```python
from build123d import *

# Parameters (mm, degrees)
SKETCH_1_R          = 2.9
EXTRUDE_3_DEPTH     = 1
EXTRUDE_6_DEPTH     = 47
CUT_EXTRUDE_START   = -1.3
CUT_EXTRUDE_1_DEPTH = 1.3
CUT_EXTRUDE_START_2 = -1.5
SKETCH_6_W          = 2.2
SKETCH_6_H          = 2.6
CUT_EXTRUDE_2_DEPTH = 1.5


with BuildPart() as part:
    # Эскиз1 → Бобышка-Вытянуть3 (new body)
    with BuildSketch(Plane(origin=(0, 0, 0), x_dir=(1, 0, 0), z_dir=(0, 1, 0))):
        with BuildLine():
            Line((-11.72321672, 11.668784432), (-11.72321672, 27.268784432))
            ThreePointArc((-11.72321672, 27.268784432), (-11.137430283, 28.682997994), (-9.72321672, 29.268784432))
            Line((-9.72321672, 29.268784432), (11.27678328, 29.268784432))
            ThreePointArc((11.27678328, 29.268784432), (12.690996842, 28.682997994), (13.27678328, 27.268784432))
            Line((13.27678328, 27.268784432), (13.27678328, 11.668784432))
            ThreePointArc((13.27678328, 11.668784432), (12.690996842, 10.254570869), (11.27678328, 9.668784432))
            Line((11.27678328, 9.668784432), (9.27678328, 9.668784432))
            Line((9.27678328, 9.668784432), (-9.72321672, 9.668784432))
            ThreePointArc((-9.72321672, 9.668784432), (-11.137430283, 10.254570869), (-11.72321672, 11.668784432))
        make_face()
        with Locations(Location((5.02678328, 15.968784432, 0), (0, 0, 270))):
            Circle(SKETCH_1_R, mode=Mode.SUBTRACT)
        with BuildLine():
            Line((-1.45321672, 26.968784432), (5.00678328, 26.968784432))
            ThreePointArc((5.00678328, 26.968784432), (6.187651604, 26.479652756), (6.67678328, 25.298784432))
            Line((6.67678328, 25.298784432), (6.67678328, 24.638784432))
            ThreePointArc((6.67678328, 24.638784432), (6.187651604, 23.457916107), (5.00678328, 22.968784432))
            Line((5.00678328, 22.968784432), (-1.45321672, 22.968784432))
            ThreePointArc((-1.45321672, 22.968784432), (-2.634085045, 23.457916107), (-3.12321672, 24.638784432))
            Line((-3.12321672, 24.638784432), (-3.12321672, 25.298784432))
            ThreePointArc((-3.12321672, 25.298784432), (-2.634085045, 26.479652756), (-1.45321672, 26.968784432))
        make_face(mode=Mode.SUBTRACT)
    extrude(amount=EXTRUDE_3_DEPTH)

    # Эскиз3 → Бобышка-Вытянуть6 (add)
    with BuildSketch(Plane(origin=(0, 1, 0), x_dir=(1, 0, 0), z_dir=(0, 1, 0))):
        with BuildLine():
            Line((-11.72321672, 27.268784432), (-11.72321672, 11.668784432))
            ThreePointArc((-11.72321672, 11.668784432), (-11.137430283, 10.254570869), (-9.72321672, 9.668784432))
            Line((-9.72321672, 9.668784432), (11.27678328, 9.668784432))
            ThreePointArc((11.27678328, 9.668784432), (12.690996842, 10.254570869), (13.27678328, 11.668784432))
            Line((13.27678328, 11.668784432), (13.27678328, 27.268784432))
            ThreePointArc((13.27678328, 27.268784432), (12.690996842, 28.682997994), (11.27678328, 29.268784432))
            Line((11.27678328, 29.268784432), (-9.72321672, 29.268784432))
            ThreePointArc((-9.72321672, 29.268784432), (-11.137430283, 28.682997994), (-11.72321672, 27.268784432))
        make_face()
        with BuildLine():
            Line((12.27678328, 14.968784432), (9.27678328, 14.968784432))
            Line((9.27678328, 14.968784432), (9.27678328, 13.818784432))
            Line((9.27678328, 13.818784432), (10.57678328, 13.818784432))
            Line((10.57678328, 13.818784432), (10.57678328, 11.318784432))
            Line((10.57678328, 11.318784432), (9.27678328, 11.318784432))
            Line((9.27678328, 11.318784432), (9.27678328, 10.668784432))
            Line((9.27678328, 10.668784432), (-7.72321672, 10.668784432))
            Line((-7.72321672, 10.668784432), (-7.72321672, 11.318784432))
            Line((-7.72321672, 11.318784432), (-9.02321672, 11.318784432))
            Line((-9.02321672, 11.318784432), (-9.02321672, 13.818784432))
            Line((-9.02321672, 13.818784432), (-7.72321672, 13.818784432))
            Line((-7.72321672, 13.818784432), (-7.72321672, 14.968784432))
            Line((-7.72321672, 14.968784432), (-10.72321672, 14.968784432))
            Line((-10.72321672, 14.968784432), (-10.72321672, 20.068784432))
            Line((-10.72321672, 20.068784432), (-7.22321672, 20.068784432))
            Line((-7.22321672, 20.068784432), (-7.22321672, 21.068784432))
            Line((-7.22321672, 21.068784432), (-8.52321672, 21.068784432))
            Line((-8.52321672, 21.068784432), (-8.52321672, 23.668784432))
            Line((-8.52321672, 23.668784432), (-7.22321672, 23.668784432))
            Line((-7.22321672, 23.668784432), (-7.22321672, 24.668784432))
            Line((-7.22321672, 24.668784432), (-10.72321672, 24.668784432))
            Line((-10.72321672, 24.668784432), (-10.72321672, 27.268784432))
            ThreePointArc((-10.72321672, 27.268784432), (-10.430323502, 27.975891213), (-9.72321672, 28.268784432))
            Line((-9.72321672, 28.268784432), (11.27678328, 28.268784432))
            ThreePointArc((11.27678328, 28.268784432), (11.983890061, 27.975891213), (12.27678328, 27.268784432))
            Line((12.27678328, 27.268784432), (12.27678328, 24.668784432))
            Line((12.27678328, 24.668784432), (8.77678328, 24.668784432))
            Line((8.77678328, 24.668784432), (8.77678328, 23.668784432))
            Line((8.77678328, 23.668784432), (10.07678328, 23.668784432))
            Line((10.07678328, 23.668784432), (10.07678328, 21.068784432))
            Line((10.07678328, 21.068784432), (8.77678328, 21.068784432))
            Line((8.77678328, 21.068784432), (8.77678328, 20.068784432))
            Line((8.77678328, 20.068784432), (12.27678328, 20.068784432))
            Line((12.27678328, 20.068784432), (12.27678328, 14.968784432))
        make_face(mode=Mode.SUBTRACT)
    extrude(amount=EXTRUDE_6_DEPTH)

    # Эскиз5 → Вырез-Вытянуть1 (cut)
    with BuildSketch(Plane(origin=(0, 48, 0), x_dir=(1, 0, 0), z_dir=(0, 1, 0)).offset(CUT_EXTRUDE_START)):
        with BuildLine():
            Line((-9.72321672, 28.268784432), (11.27678328, 28.268784432))
            ThreePointArc((11.27678328, 28.268784432), (11.983890061, 27.975891213), (12.27678328, 27.268784432))
            Line((12.27678328, 27.268784432), (12.27678328, 11.668784432))
            ThreePointArc((12.27678328, 11.668784432), (11.983890061, 10.961677651), (11.27678328, 10.668784432))
            Line((11.27678328, 10.668784432), (-9.72321672, 10.668784432))
            ThreePointArc((-9.72321672, 10.668784432), (-10.430323502, 10.961677651), (-10.72321672, 11.668784432))
            Line((-10.72321672, 11.668784432), (-10.72321672, 27.268784432))
            ThreePointArc((-10.72321672, 27.268784432), (-10.430323502, 27.975891213), (-9.72321672, 28.268784432))
        make_face()
    extrude(amount=CUT_EXTRUDE_1_DEPTH, mode=Mode.SUBTRACT)

    # Эскиз6 → Вырез-Вытянуть2 (cut)
    with BuildSketch(Plane(origin=(0, 46.7, 0), x_dir=(1, 0, 0), z_dir=(0, 1, 0)).offset(CUT_EXTRUDE_START_2)):
        with Locations((-9.62321672, 22.368784432)):
            Rectangle(SKETCH_6_W, SKETCH_6_H)
        with Locations((11.17678328, 22.368784432)):
            Rectangle(SKETCH_6_W, SKETCH_6_H)
        with BuildLine():
            Line((10.57678328, 13.818784432), (10.57678328, 11.318784432))
            Line((10.57678328, 11.318784432), (12.213532979, 11.318784432))
            ThreePointArc((12.213532979, 11.318784432), (12.260843669, 11.490949817), (12.27678328, 11.668784432))
            Line((12.27678328, 11.668784432), (12.27678328, 13.818784432))
            Line((12.27678328, 13.818784432), (10.57678328, 13.818784432))
        make_face()
        with BuildLine():
            Line((-9.02321672, 13.818784432), (-10.72321672, 13.818784432))
            Line((-10.72321672, 13.818784432), (-10.72321672, 11.668784432))
            ThreePointArc((-10.72321672, 11.668784432), (-10.70727711, 11.490949817), (-10.65996642, 11.318784432))
            Line((-10.65996642, 11.318784432), (-9.02321672, 11.318784432))
            Line((-9.02321672, 11.318784432), (-9.02321672, 13.818784432))
        make_face()
    extrude(amount=CUT_EXTRUDE_2_DEPTH, mode=Mode.SUBTRACT)


solid = part.part
```
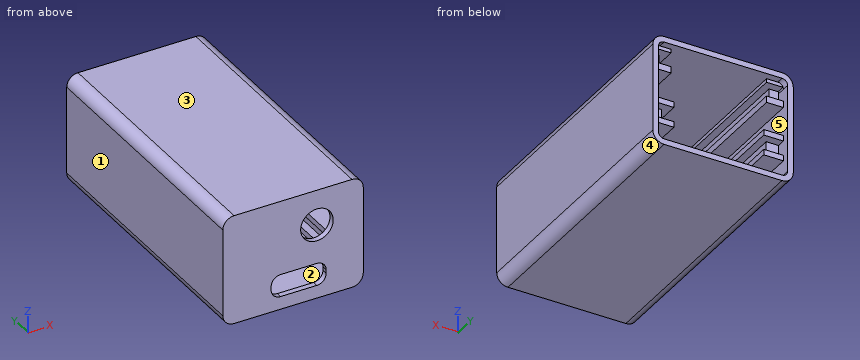
For this review, take the finished solid that the model builds, in its own axes (mm). Face numbers are marked on the shaded views. A direction names the side the tool comes from. Round coordinates to 2 decimals unless told otherwise and drop trailing zeros. Write each loop counter-clockwise with the first axis right and the second up, starting at its lowest first coordinate (ties: lowest second). Pieces come first, ordered by that corner, then holes. Notation, with made-up numbers: M 54,88.25 L 89,88.25 A20 cw 89,107.25 Z; hole C 76.25,77 d4. An arc over 180 degrees is marked long. One line per item, written item: value. Start each with the question number.
(1) The part is to be moulded in two halves that separate along X. For the marked faces 3, 4 and 5, say which applies: released by +X, released by -X, zero draft, split by the parting line, or undercut.
(2) We need section B-B (z = -15.75). Give the boundary of the cut face in (x, y).
(3) We need section D-D (z = -22.25). Give the boundary of the cut face in (x, y), and give its area (3 significant figures).
(4) Insertion check: pin 1 (2 mm diameter, centred on x = -8, z = -15.5, fed in from -Y); pin 2 (1.8 mm diameter, centred on x = -9, z = -23, fed in from +Y). Each pin has a flat end and moves straight along its axis. Give the tip position at first contact, or say it passes through.
(5) We need section A-A (x = 0). Give the boundary of the cut face in (y, z).
(6) Wall thickness on line 1 (Z direction, x = 11.25, y = 16); line 2 (Z direction, x = -8, y = 15); line 3 (Z direction, x = 10.25, y = 18.5): over which ranges is each line inside the solid? List them lowest first.
(7) Machinability: for the marked faces 1 and 2, which of the approach directions +Z, -Z, +X, -X, +Y, -Y give a long, thin tool a straight path to every point of the face, cutting with its end or side? Answer none if there is none.
(8) We need section C-C (x = 4.5). Give the boundary of the cut face in (y, z).
Result:
1. face 3: zero draft
1. face 4: released by +X
1. face 5: undercut
2. outline: M -11.72,0 L 2.14,0 L 2.14,1 L -10.72,1 L -10.72,48 L -11.72,48 Z; M 7.92,0 L 13.28,0 L 13.28,48 L 12.28,48 L 12.28,1 L 7.92,1 Z
3. outline: M -11.72,0 L 13.28,0 L 13.28,48 L 12.28,48 L 12.28,45.2 L 10.08,45.2 L 10.08,1 L -8.52,1 L -8.52,45.2 L -10.72,45.2 L -10.72,48 L -11.72,48 Z
3. area: 313 mm²
4. pin 1: y = 0
4. pin 2: y = 46.7
5. outline: M 0,-29.27 L 48,-29.27 L 48,-28.27 L 1,-28.27 L 1,-26.97 L 0,-26.97 Z; M 0,-22.97 L 1,-22.97 L 1,-10.67 L 48,-10.67 L 48,-9.67 L 0,-9.67 Z
6. line 1: -29.27 to -28.27, -24.67 to -20.07, -14.97 to -9.67
6. line 2: -29.27 to -28.27, -24.67 to -23.67, -21.07 to -20.07, -14.97 to -13.82, -11.32 to -9.67
6. line 3: -29.27 to -28.27, -24.67 to -20.07, -14.97 to -13.82, -11.32 to -9.67
7. face 1: +Z, -Z, -X, +Y, -Y
7. face 2: +Y
8. outline: M 0,-29.27 L 48,-29.27 L 48,-28.27 L 1,-28.27 L 1,-26.97 L 0,-26.97 Z; M 0,-22.97 L 1,-22.97 L 1,-18.82 L 0,-18.82 Z; M 0,-13.12 L 1,-13.12 L 1,-10.67 L 48,-10.67 L 48,-9.67 L 0,-9.67 Z
